Could you check a few things on this model? Use its own coordinates, in mm. A direction names the side the tool comes from. Give positions to 0.01 mm unless a question says otherwise; leave off trailing zeros. Order: outer loops, then holes, each group sorted by start corner. A loop starts at its lowest first (then second) coordinate and runs counter-clockwise, first axis right, second up. Notation, with made-up numbers: M 51,5 L 74,5 A31 cw 74,35 Z; hole C -16.5,-17.75 d5. An arc over 180 degrees is marked long. Answer in a Markdown table with one row per item. Add a question column.
```python
from build123d import *

# Parameters (mm, degrees)
F0_R     = 1.65
F0_R_2   = 1.55
F0_W     = 15
F0_H     = 29
F0_W_2   = 33
F1_DEPTH = 3
F2_W     = 182.5
F2_H     = 38
F2_W_2   = 178
F2_H_2   = 34
F3_DEPTH = 60
F4_R     = 2.1
F5_DEPTH = 25
F6_R     = 2.1
F7_DEPTH = 25
F8_W     = 60.5
F8_H     = 38
F9_DEPTH = 2
F10_SIZE = 5


with BuildPart() as f1:
    # F0 (on Front) → F1 (new body)
    with BuildSketch(Plane.XZ):
        with BuildLine():
            Line((86, 72), (-86, 72))
            ThreePointArc((-86, 72), (-89.5355339059, 70.5355339059), (-91, 67))
            Line((-91, 67), (-91, 5))
            ThreePointArc((-91, 5), (-89.5355339059, 1.4644660941), (-86, 0))
            Line((-86, 0), (86, 0))
            ThreePointArc((86, 0), (89.5355339059, 1.4644660941), (91, 5))
            Line((91, 5), (91, 67))
            ThreePointArc((91, 67), (89.5355339059, 70.5355339059), (86, 72))
        make_face()
        with Locations((-85, 6)):
            Circle(F0_R, mode=Mode.SUBTRACT)
        with Locations((0, 6)):
            Circle(F0_R, mode=Mode.SUBTRACT)
        with Locations((85, 6)):
            Circle(F0_R, mode=Mode.SUBTRACT)
        with Locations((72.5, 17.2)):
            Circle(F0_R_2, mode=Mode.SUBTRACT)
        with Locations((44.5, 36)):
            Rectangle(F0_W, F0_H, mode=Mode.SUBTRACT)
        with Locations((72.5, 36)):
            Rectangle(F0_W_2, F0_H, mode=Mode.SUBTRACT)
        with Locations((-85, 66)):
            Circle(F0_R, mode=Mode.SUBTRACT)
        with Locations((0, 66)):
            Circle(F0_R, mode=Mode.SUBTRACT)
        with Locations((72.5, 54.8)):
            Circle(F0_R_2, mode=Mode.SUBTRACT)
        with Locations((85, 66)):
            Circle(F0_R, mode=Mode.SUBTRACT)
    extrude(amount=F1_DEPTH)

    # F2 (on face) → F3 (join)
    with BuildSketch(Plane.XZ):
        with Locations((0.25, 36)):
            Rectangle(F2_W, F2_H)
        with Locations((0, 36)):
            Rectangle(F2_W_2, F2_H_2, mode=Mode.SUBTRACT)
    extrude(amount=-F3_DEPTH)

    # F4 (on face) → F5 (cut)
    with BuildSketch(Plane(origin=(0, 0, 17), x_dir=(1, 0, 0), z_dir=(0, 0, -1))):
        with Locations((-52.5, -47.5)):
            Circle(F4_R)
        with Locations((-2.5, -47.5)):
            Circle(F4_R)
    extrude(amount=-F5_DEPTH, mode=Mode.SUBTRACT)

    # F6 (on face) → F7 (cut)
    with BuildSketch(Plane(origin=(-91, 0, 0), x_dir=(0, -1, 0), z_dir=(-1, 0, 0))):
        with Locations((-47.5, 33.5)):
            Circle(F6_R)
    extrude(amount=-F7_DEPTH, mode=Mode.SUBTRACT)

    # F8 (on face) → F9 (join)
    with BuildSketch(Plane(origin=(0, 60, 0), x_dir=(-1, 0, 0), z_dir=(0, 1, 0))):
        with Locations((-61.25, 36)):
            Rectangle(F8_W, F8_H)
    extrude(amount=F9_DEPTH)

    # F10
    f10_edges = [f1.edges().sort_by_distance(p)[0] for p in [
        (89, 60, 36),
        (60, 60, 53),
        (60, 60, 19),
    ]]
    chamfer(f10_edges, length=F10_SIZE)


solid = f1.part
```
1. Suppose I cut it at D-D on y = 47.5. List the corners of the cut face in (x, z) for me.
2. Will these pins go through, and if not, where does the flat tip stop? P1, Ø0.5, axis at x = 72.5, z = 54, coming from the -Y side; P2, Ø1, axis at x = -51.5, y = 4.5, coming from the -Z side; P3, Ø2, axis at x = 65.5, y = 14, coming from the +Z side.
3. Suppose I cut it at A-A on x = -52.5. List the corners of the cut face in (y, z) for me, plus the area to 3 significant figures.
4. Thinking about a two-plate mould opening in Z: for faces 1 (the cylindrical face through (83.35, -1.48, 6.07)), 2 (the flat face through (91.5, 31, 36)), 3 (the cylindrical face through (-89, -1, 71)), 4 (the flat face through (2, 31, 17)), which applies, pulls with the +Z half, pulls with the -Z half, needs draft (parallel to the pull), parting line crosses it, or undercut?
5. If I drill on line 1 along X through (y, z) = (19, 20); line 2 along Z through (x, y) = (-67, 31); line 3 along Z through (x, y) = (-90.4, 47.5), over which ranges is the centre line in solid material (lowest first)? Write a range as [from, to].
6. For faces 5 (the cylindrical face through (-51.531, 49.363, 17.986)), 6 (the flat face through (89, 26, 36)), 7 (the flat face through (-1, 0, 9)), which set-ups out of +Z, -Z, +X, -X, +Y, -Y let a thin tool reach every point of the face, with its end or its side?
7. Suppose I cut it at C-C on y = 57. List the corners of the cut face in (x, z) for me.
8. Suppose I cut it at B-B on z = 33.5. List the corners of the cut face in (x, y) for me.
Findings below:
| question | item | result |
|---|---|---|
| 1 | outline | M -91,17 L -54.6,17 L -54.6,19 L -89,19 L -89,31.4 L -91,31.4 Z; M -91,35.6 L -89,35.6 L -89,53 L 89,53 L 89,19 L -0.4,19 L -0.4,17 L 91.5,17 L 91.5,55 L -91,55 Z; M -50.4,17 L -4.6,17 L -4.6,19 L -50.4,19 Z |
| 2 | P1 | y = 0 |
| 2 | P2 | z = 17 |
| 2 | P3 | z = 55 |
| 3 | outline | M -3,0 L 0,0 L 0,17 L 45.4,17 L 45.4,19 L 0,19 L 0,53 L 60,53 L 60,55 L 0,55 L 0,72 L -3,72 Z; M 49.6,17 L 60,17 L 60,19 L 49.6,19 Z |
| 3 | area | 448 mm2 |
| 4 | face 1 | undercut |
| 4 | face 2 | needs draft |
| 4 | face 3 | pulls with the +Z half |
| 4 | face 4 | pulls with the -Z half |
| 5 | line 1 | [-91, -89], [89, 91.5] |
| 5 | line 2 | [17, 19], [53, 55] |
| 5 | line 3 | [17, 31.4], [35.6, 55] |
| 6 | face 5 | -Z |
| 6 | face 6 | none |
| 6 | face 7 | -Z, +X, -X, +Y |
| 7 | outline | M -91,17 L 91.5,17 L 91.5,55 L -91,55 Z; hole M -89,19 L 31,19 L 31,21 L 87,21 L 87,51 L 31,51 L 31,53 L -89,53 Z |
| 8 | outline | M -91,-3 L 37,-3 L 37,0 L -89,0 L -89,45.4 L -91,45.4 Z; M -91,49.6 L -89,49.6 L -89,60 L -91,60 Z; M 31,60 L 84,60 L 89,55 L 89,-3 L 91,-3 L 91,0 L 91.5,0 L 91.5,62 L 31,62 Z; M 52,-3 L 56,-3 L 56,0 L 52,0 Z |
